Geometry check sheet. Reference: the model listing, model coordinates, mm. Face numbers are marked on the shaded views. A direction names the side the tool comes from. Coordinates: 2 decimals unless noted, no trailing zeros. Loops run counter-clockwise (first coordinate to the right, second up) from the corner with the lowest first, then second, coordinate; pieces in that order, holes last.
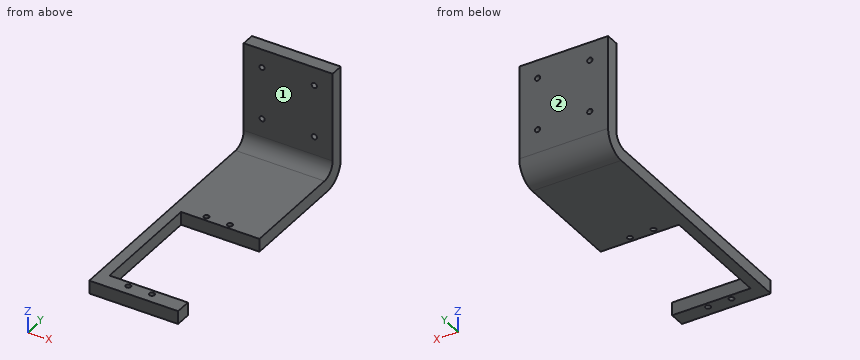
from build123d import *

# Parameters (mm, degrees)
SKETCH1_R           = 1
BOSS_EXTRUDE1_DEPTH = 5
SKETCH2_W           = 34
SKETCH2_H           = 44
SKETCH2_R           = 1
BOSS_EXTRUDE2_DEPTH = 5
FILLET1_R           = 8
FILLET3_R           = 5


with BuildPart() as part:
    # Sketch1 → Boss-Extrude1 (new body)
    with BuildSketch(Plane.XY):
        Polygon((-17, 67), (-17, -28), (17, -28), (17, -22), (13, -22), (-13, -22), (-13, -21.411764706), (-13, 22), (13, 22), (17, 22), (17, 67), align=None)
        with Locations((-4.5, -24)):
            Circle(SKETCH1_R, mode=Mode.SUBTRACT)
        with Locations((4.5, -24)):
            Circle(SKETCH1_R, mode=Mode.SUBTRACT)
        with Locations((-4.5, 24)):
            Circle(SKETCH1_R, mode=Mode.SUBTRACT)
        with Locations((4.5, 24)):
            Circle(SKETCH1_R, mode=Mode.SUBTRACT)
    extrude(amount=BOSS_EXTRUDE1_DEPTH)

    # Sketch2 → Boss-Extrude2 (add)
    with BuildSketch(Plane(origin=(0, 67, 0), x_dir=(1, 0, 0), z_dir=(0, 1, 0))):
        with Locations((0, -22)):
            Rectangle(SKETCH2_W, SKETCH2_H)
        with Locations((-10, -17)):
            Circle(SKETCH2_R, mode=Mode.SUBTRACT)
        with Locations((10, -17)):
            Circle(SKETCH2_R, mode=Mode.SUBTRACT)
        with Locations((10, -37)):
            Circle(SKETCH2_R, mode=Mode.SUBTRACT)
        with Locations((-10, -37)):
            Circle(SKETCH2_R, mode=Mode.SUBTRACT)
    extrude(amount=BOSS_EXTRUDE2_DEPTH)

    # Fillet1
    fillet1_edges = [part.edges().sort_by_distance(p)[0] for p in [
        (0, 72, 0),
    ]]
    fillet(fillet1_edges, radius=FILLET1_R)

    # Fillet3
    fillet3_edges = [part.edges().sort_by_distance(p)[0] for p in [
        (0, 67, 5),
    ]]
    fillet(fillet3_edges, radius=FILLET3_R)


solid = part.part
(1) Sectioned sample at D-D on x = 4.5. Record the cut outline in (y, z), and give its area (3 significant figures).
Findings:
outline: (-28, 0) - (-25, 0) - (-25, 5) - (-28, 5) - close; (-23, 0) - (-22, 0) - (-22, 5) - (-23, 5) - close; (22, 0) - (23, 0) - (23, 5) - (22, 5) - close; (25, 0) - (64, 0) arc R8 ccw to (72, 8) - (72, 44) - (67, 44) - (67, 10) arc R5 cw to (62, 5) - (25, 5) - close
area: 447 mm2
(2) Sectioned sample at A-A on y = 24. Record the cut outline in (x, z).
Findings:
outline: (-17, 0) - (-5.5, 0) - (-5.5, 5) - (-17, 5) - close; (-3.5, 0) - (3.5, 0) - (3.5, 5) - (-3.5, 5) - close; (5.5, 0) - (17, 0) - (17, 5) - (5.5, 5) - close
(3) Gauge pin test, flat ends, axial feed: pin 1 Ø2.5 at (x, y) = (4.5, -24) entering from +Z; pin 2 Ø1 at (x, z) = (-6, 24) entering from -Y; pin 3 Ø8 at (x, y) = (-8, 61) entering from +Z. Record the tip position at first contact, or that the pin passes through.
Findings:
pin 1: stops at z = 5
pin 2: stops at y = 67
pin 3: stops at z = 6
(4) Scan lines: L1, parallel to X at y = 68, z = 37; L2, parallel to Z at x = 10, y = 69.2; L3, parallel to Z at x = 10, y = 70. Record each from-to range of solid material in increasing order.
Findings:
L1: x = -17 to -11, -9 to 9, 11 to 17
L2: z = 1.92 to 16, 18 to 36, 38 to 44
L3: z = 2.71 to 16, 18 to 36, 38 to 44
(5) Access from +Z, -Z, +X, -X, +Y, -Y to the whole of each face (thin tool, end or side, straight path). Record for the marked faces 1 and 2.
Findings:
face 1: +Z, +X, -X, -Y
face 2: +Z, -Z, +X, -X, +Y
(6) Sectioned sample at C-C on x = -7. Record the cut outline in (y, z), and give its area (3 significant figures).
Findings:
outline: (-28, 0) - (-22, 0) - (-22, 5) - (-28, 5) - close; (22, 0) - (64, 0) arc R8 ccw to (72, 8) - (72, 44) - (67, 44) - (67, 10) arc R5 cw to (62, 5) - (22, 5) - close
area: 467 mm2
(7) Sectioned sample at B-B on z = 37. Record the cut outline in (x, y).
Findings:
outline: (-17, 67) - (-11, 67) - (-11, 72) - (-17, 72) - close; (-9, 67) - (9, 67) - (9, 72) - (-9, 72) - close; (11, 67) - (17, 67) - (17, 72) - (11, 72) - close
